from build123d import *

# Parameters (mm, degrees)
SKETCH_1_W      = 12
SKETCH_1_H      = 11
EXTRUDE_1_DEPTH = 20
SKETCH_2_R      = 1.5
EXTRUDE_2_DEPTH = 1
SKETCH_3_R      = 0.75
EXTRUDE_3_DEPTH = 4.5


with BuildPart() as part:
    # ｽｹｯﾁ1 → ﾎﾞｽ - 押し出し1 (new body)
    with BuildSketch(Plane.XY):
        Rectangle(SKETCH_1_W, SKETCH_1_H)
    extrude(amount=EXTRUDE_1_DEPTH)

    # ｽｹｯﾁ2 → ﾎﾞｽ - 押し出し2 (add)
    with BuildSketch(Plane(origin=(0, 0, 0), x_dir=(-1, 0, 0), z_dir=(0, 0, -1))):
        Circle(SKETCH_2_R)
    extrude(amount=EXTRUDE_2_DEPTH)

    # ｽｹｯﾁ3 → ﾎﾞｽ - 押し出し3 (add)
    with BuildSketch(Plane(origin=(0, 0, 0), x_dir=(-1, 0, 0), z_dir=(0, 0, -1))):
        Circle(SKETCH_3_R)
    extrude(amount=EXTRUDE_3_DEPTH)


solid = part.part
Build history of the part. All positions in model axes, mm. A direction names the side the tool comes from. Round coordinates to 2 decimals unless told otherwise and drop trailing zeros. Write each loop counter-clockwise with the first axis right and the second up, starting at its lowest first coordinate (ties: lowest second). Pieces come first, ordered by that corner, then holes. Notation, with made-up numbers: M -8.5,81 L 30.5,81 A8 ccw 30.5,93 Z; hole C 85,-23.75 d1. An arc over 180 degrees is marked long. Use CSV: the item, a comma, the result in double quotes.
1. Tool access for faces 1 (the face through (1, 0, -1)), 2 (the face through (6, 0, 10)): list every direction of +Z, -Z, +X, -X, +Y, -Y with a clear straight run to the whole face (end or side of a thin tool).
Reply:
face 1,"-Z"
face 2,"+Z, -Z, +X, +Y, -Y"
2. Saw through at C-C (z = -0.75). Give the cut face in (x, y), plus the area to 3 significant figures.
Reply:
outline,"C 0,0 d3"
area,"7.07 mm²"
3. Saw through at D-D (y = 1.25). Give the cut face in (x, z).
Reply:
outline,"M -6,0 L -0.83,0 L -0.83,-1 L 0.83,-1 L 0.83,0 L 6,0 L 6,20 L -6,20 Z"
4. Saw through at A-A (y = 0). Give the cut face in (x, z).
Reply:
outline,"M -6,0 L -1.5,0 L -1.5,-1 L -0.75,-1 L -0.75,-4.5 L 0.75,-4.5 L 0.75,-1 L 1.5,-1 L 1.5,0 L 6,0 L 6,20 L -6,20 Z"
5. Wall check: probe 1 along Z at (x, y) = (-3.75, 3); probe 2 along Z at (x, y) = (0.75, -1.25). Give the ranges that are in metal, low to high. Write a range as from..to.
Reply:
probe 1,"z = 0..20"
probe 2,"z = -1..20"
6. Saw through at B-B (x = 0). Give the cut face in (y, z).
Reply:
outline,"M -5.5,0 L -1.5,0 L -1.5,-1 L -0.75,-1 L -0.75,-4.5 L 0.75,-4.5 L 0.75,-1 L 1.5,-1 L 1.5,0 L 5.5,0 L 5.5,20 L -5.5,20 Z"
7. Flat gauge pins, fed straight in: pin 1 (3 mm diameter, centred on x = 1.5, y = 4, fed in from -Z); pin 2 (3.5 mm diameter, centred on x = 2, y = 2.5, fed in from -Z); pin 3 (6 mm diameter, centred on x = -3, y = -1.5, fed in from -Z). Where does each tip first touch, or does it go through?
Reply:
pin 1,"stops at z = 0"
pin 2,"stops at z = -1"
pin 3,"stops at z = -4.5"
